from build123d import *

# Parameters (mm, degrees)
SKETCH1_W                     = 80
SKETCH1_H                     = 35
RECTANGLE_BLOCK_EXTRUDE_DEPTH = 45
HOLLOW_OUT_BLOCK_CUT_DEPTH    = 81
OPEN_CORNER_CUT_DEPTH         = 81
TOP_CUTS_REACH                = 37
SKETCH15_R                    = 4
CIRCLE_CUT_ON_FRONT_REACH     = 12
SKETCH18_R                    = 4
RECTANGLE_CUT_ON_BACK_DEPTH   = 5
CUT_EXTRUDE17_DEPTH           = 81
SKETCH25_W                    = 40
SKETCH25_H                    = 3
SKETCH25_H_2                  = 17
CUT_EXTRUDE18_DEPTH           = 10
BOSS_EXTRUDE6_DEPTH           = 5


with BuildPart() as part:
    # Sketch1 → Rectangle Block Extrude (new body)
    with BuildSketch(Plane.XY):
        Rectangle(SKETCH1_W, SKETCH1_H)
    extrude(amount=RECTANGLE_BLOCK_EXTRUDE_DEPTH)

    # Sketch11 → Hollow Out Block Cut (cut, through all)
    with BuildSketch(Plane.ZY.offset(40)):
        with BuildLine():
            Line((8, 12.5), (37, 12.5))
            ThreePointArc((37, 12.5), (39.121320344, 11.621320344), (40, 9.5))
            Line((40, 9.5), (40, -9.5))
            ThreePointArc((40, -9.5), (39.121320344, -11.621320344), (37, -12.5))
            Line((37, -12.5), (8, -12.5))
            ThreePointArc((8, -12.5), (5.878679656, -11.621320344), (5, -9.5))
            Line((5, -9.5), (5, 9.5))
            ThreePointArc((5, 9.5), (5.878679656, 11.621320344), (8, 12.5))
        make_face()
    extrude(amount=-HOLLOW_OUT_BLOCK_CUT_DEPTH, mode=Mode.SUBTRACT)

    # Sketch12 → Open Corner Cut (cut, through all)
    with BuildSketch(Plane.ZY.offset(40)):
        with BuildLine():
            Line((35, 17.5), (35, 12.5))
            Line((35, 12.5), (37, 12.5))
            ThreePointArc((37, 12.5), (39.121320344, 11.621320344), (40, 9.5))
            Line((40, 9.5), (40, 2.5))
            Line((40, 2.5), (45, 2.5))
            Line((45, 2.5), (45, 17.5))
            Line((45, 17.5), (35, 17.5))
        make_face()
    extrude(amount=-OPEN_CORNER_CUT_DEPTH, mode=Mode.SUBTRACT)

    # Sketch15 → Top Cuts (cut, up to next)
    with BuildSketch(Plane(origin=(0, 17.5, 0), x_dir=(1, 0, 0), z_dir=(0, 1, 0)), mode=Mode.PRIVATE) as top_cuts_sk1:
        with BuildLine():
            Line((17, -8), (-17, -8))
            ThreePointArc((-17, -8), (-19.121320344, -8.878679656), (-20, -11))
            Line((-20, -11), (-20, -35))
            Line((-20, -35), (20, -35))
            Line((20, -35), (20, -11))
            ThreePointArc((20, -11), (19.121320344, -8.878679656), (17, -8))
        make_face()
    top_cuts_tool1 = extrude(top_cuts_sk1.sketch, amount=-TOP_CUTS_REACH, mode=Mode.PRIVATE) & part.part
    add(top_cuts_tool1.solids().sort_by_distance((0, 17.5, 21.546053))[0], mode=Mode.SUBTRACT)
    # Sketch15 → Top Cuts (cut, up to next)
    with BuildSketch(Plane(origin=(0, 17.5, 0), x_dir=(1, 0, 0), z_dir=(0, 1, 0)), mode=Mode.PRIVATE) as top_cuts_sk2:
        with Locations((-30, -23)):
            Circle(SKETCH15_R)
    top_cuts_tool2 = extrude(top_cuts_sk2.sketch, amount=-TOP_CUTS_REACH, mode=Mode.PRIVATE) & part.part
    add(top_cuts_tool2.solids().sort_by_distance((-30, 17.5, 23))[0], mode=Mode.SUBTRACT)
    # Sketch15 → Top Cuts (cut, up to next)
    with BuildSketch(Plane(origin=(0, 17.5, 0), x_dir=(1, 0, 0), z_dir=(0, 1, 0)), mode=Mode.PRIVATE) as top_cuts_sk3:
        with Locations((30, -23)):
            Circle(SKETCH15_R)
    top_cuts_tool3 = extrude(top_cuts_sk3.sketch, amount=-TOP_CUTS_REACH, mode=Mode.PRIVATE) & part.part
    add(top_cuts_tool3.solids().sort_by_distance((30, 17.5, 23))[0], mode=Mode.SUBTRACT)

    # Sketch18 → Circle Cut on Front (cut, up to next)
    with BuildSketch(Plane.XY.offset(35), mode=Mode.PRIVATE) as circle_cut_on_front_sk1:
        with Locations((-30, -5.5)):
            Circle(SKETCH18_R)
    circle_cut_on_front_tool1 = extrude(circle_cut_on_front_sk1.sketch, amount=CIRCLE_CUT_ON_FRONT_REACH, mode=Mode.PRIVATE) & part.part
    add(circle_cut_on_front_tool1.solids().sort_by_distance((-30, -5.5, 35))[0], mode=Mode.SUBTRACT)
    # Sketch18 → Circle Cut on Front (cut, up to next)
    with BuildSketch(Plane.XY.offset(35), mode=Mode.PRIVATE) as circle_cut_on_front_sk2:
        with Locations((30, -5.5)):
            Circle(SKETCH18_R)
    circle_cut_on_front_tool2 = extrude(circle_cut_on_front_sk2.sketch, amount=CIRCLE_CUT_ON_FRONT_REACH, mode=Mode.PRIVATE) & part.part
    add(circle_cut_on_front_tool2.solids().sort_by_distance((30, -5.5, 35))[0], mode=Mode.SUBTRACT)

    # Sketch23 → Rectangle Cut on Back (cut)
    with BuildSketch(Plane(origin=(0, 0, 0), x_dir=(-1, 0, 0), z_dir=(0, 0, -1))):
        with BuildLine():
            Line((22, 5.5), (-22, 5.5))
            ThreePointArc((-22, 5.5), (-24.121320344, 4.621320344), (-25, 2.5))
            Line((-25, 2.5), (-25, -2.5))
            ThreePointArc((-25, -2.5), (-24.121320344, -4.621320344), (-22, -5.5))
            Line((-22, -5.5), (22, -5.5))
            ThreePointArc((22, -5.5), (24.121320344, -4.621320344), (25, -2.5))
            Line((25, -2.5), (25, 2.5))
            ThreePointArc((25, 2.5), (24.121320344, 4.621320344), (22, 5.5))
        make_face()
    extrude(amount=-RECTANGLE_CUT_ON_BACK_DEPTH, mode=Mode.SUBTRACT)

    # Sketch24 → Cut-Extrude17 (cut, through all)
    with BuildSketch(Plane.ZY.offset(40)):
        with BuildLine():
            Line((3, -17.5), (0, -17.5))
            Line((0, -17.5), (0, -14.5))
            ThreePointArc((0, -14.5), (0.878679656, -16.621320344), (3, -17.5))
        make_face()
        with BuildLine():
            Line((0, 14.5), (0, 17.5))
            Line((0, 17.5), (3, 17.5))
            ThreePointArc((3, 17.5), (0.878679656, 16.621320344), (0, 14.5))
        make_face()
        with BuildLine():
            Line((42, -17.5), (45, -17.5))
            Line((45, -17.5), (45, -14.5))
            ThreePointArc((45, -14.5), (44.121320344, -16.621320344), (42, -17.5))
        make_face()
    extrude(amount=-CUT_EXTRUDE17_DEPTH, mode=Mode.SUBTRACT)

    # Sketch25 → Cut-Extrude18 (cut)
    with BuildSketch(Plane.XY.offset(45)):
        with Locations((0, -16)):
            Rectangle(SKETCH25_W, SKETCH25_H)
        with Locations((0, -6)):
            Rectangle(SKETCH25_W, SKETCH25_H_2)
    extrude(amount=-CUT_EXTRUDE18_DEPTH, mode=Mode.SUBTRACT)

    # Sketch28 → Boss-Extrude6 (add)
    with BuildSketch(Plane(origin=(0, -17.5, 0), x_dir=(-1, 0, 0), z_dir=(0, -1, 0))):
        with BuildLine():
            Line((-20, -38), (-20, -35))
            Line((-20, -35), (-17, -35))
            ThreePointArc((-17, -35), (-19.121320344, -35.878679656), (-20, -38))
        make_face()
        with BuildLine():
            Line((20, -38), (20, -35))
            Line((20, -35), (17, -35))
            ThreePointArc((17, -35), (19.121320344, -35.878679656), (20, -38))
        make_face()
    extrude(amount=-BOSS_EXTRUDE6_DEPTH)


solid = part.part
Source: CAD feature listing. Evaluate the final solid. Frame: model axes, mm. A direction names the side the tool comes from. Round coordinates to 2 decimals unless told otherwise and drop trailing zeros. Loops run counter-clockwise (first coordinate to the right, second up) from the corner with the lowest first, then second, coordinate; pieces in that order, holes last. Notation, with made-up numbers: (84.25, -4) - (111.25, -4) arc R12 cw to (111.25, 14) - close; hole circle Ø5 at (-35, 1.5). An arc over 180 degrees is marked (long way). Write item = value, one per line. Start each with the question number.
(1) Set-up query: faces 1 (the face through (-20, -7, 42)), 2 (the face through (20, 15, 23)), 3 (the face through (-29, 12.5, 18)). Return all of +Z, -Z, +X, -X, +Y, -Y with unobstructed straight access to the full face (end or side cutting, diameter ignored); none if empty.
(2) Section query D-D, the plane x = -31.5. Output: boundary loops of the cut face in (y, z), plus the area to 3 significant figures.
(3) Pin query (flat end, axial travel): pin 1 (2.5 mm diameter, centred on x = 29, y = 14, fed in from +Z); pin 2 (2 mm diameter, centred on x = 11, z = 29.5, fed in from +Y); pin 3 (5.5 mm diameter, centred on x = 28.5, z = 42.5, fed in from +Y). Return the tip coordinate at first contact, or that it passes through.
(4) Section query B-B, the plane z = 23. Output: boundary loops of the cut face in (x, y), plus the area to 3 significant figures.
(5) Section query C-C, the plane y = -4.5. Output: boundary loops of the cut face in (x, z), plus the area to 3 significant figures.
(6) Pull-direction query (Y, two-part tool) for faces 4 (the face through (40, -13, 19)), 5 (the face through (30, 2.5, 42)), 6 (the face through (0, -5.5, 2)), 7 (the face through (24.1, 4.64, 2.46)); classes: +Y half, -Y half, draft (parallel to the pull), parting line (faces both ways), or undercut.
(7) Section query A-A, the plane x = -7. Output: boundary loops of the cut face in (y, z), plus the area to 3 significant figures.
(8) Ray query, line 1 along X through (y, z) = (13.8, 23); line 2 along Y through (x, z) = (26.5, 25); line 3 along Z through (x, y) = (-16, -13.5). Return the intervals inside material, ascending. Write a range as from..to.
Conclusion:
q1.face_1 = +Z, +Y, -Y
q1.face_2 = +Z, +Y
q1.face_3 = +Z, +X, -X
q2.outline = (-17.5, 3) arc R3 ccw to (-14.5, 0) - (14.5, 0) arc R3 ccw to (17.5, 3) - (17.5, 19.29) - (12.5, 19.29) - (12.5, 8) arc R3 cw to (9.5, 5) - (-9.5, 5) arc R3 cw to (-12.5, 8) - (-12.5, 37) arc R3 cw to (-9.5, 40) - (-9.21, 40) - (-9.21, 45) - (-14.5, 45) arc R3 ccw to (-17.5, 42) - close; (-1.79, 40) - (2.5, 40) - (2.5, 45) - (-1.79, 45) - close; (12.5, 26.71) - (17.5, 26.71) - (17.5, 35) - (12.5, 35) - close
q2.area = 526 mm2
q3.pin_1 = 35
q3.pin_2 = -12.5
q3.pin_3 = 2.5
q4.outline = (-40, -17.5) - (40, -17.5) - (40, -12.5) - (-40, -12.5) - close; (-40, 12.5) - (-34, 12.5) - (-34, 17.5) - (-40, 17.5) - close; (-26, 12.5) - (-20, 12.5) - (-20, 17.5) - (-26, 17.5) - close; (20, 12.5) - (26, 12.5) - (26, 17.5) - (20, 17.5) - close; (34, 12.5) - (40, 12.5) - (40, 17.5) - (34, 17.5) - close
q4.area = 520 mm2
q5.outline = (-40, 0) - (-24.24, 0) - (-24.24, 5) - (-40, 5) - close; (-40, 40) - (-33.87, 40) - (-33.87, 45) - (-40, 45) - close; (-26.13, 40) - (-20, 40) - (-20, 45) - (-26.13, 45) - close; (20, 40) - (26.13, 40) - (26.13, 45) - (20, 45) - close; (24.24, 0) - (40, 0) - (40, 5) - (24.24, 5) - close; (33.87, 40) - (40, 40) - (40, 45) - (33.87, 45) - close
q5.area = 280 mm2
q6.face_4 = draft
q6.face_5 = +Y half
q6.face_6 = undercut
q6.face_7 = undercut
q7.outline = (-17.5, 3) arc R3 ccw to (-14.5, 0) - (-5.5, 0) - (-5.5, 5) - (-9.5, 5) arc R3 cw to (-12.5, 8) - (-12.5, 35) - (-17.5, 35) - close; (5.5, 0) - (14.5, 0) arc R3 ccw to (17.5, 3) - (17.5, 8) - (12.5, 8) arc R3 cw to (9.5, 5) - (5.5, 5) - close
q7.area = 285 mm2
q8.line_1 = -40..-34, -26..-20, 20..26, 34..40
q8.line_2 = -17.5..-12.5, 12.5..17.5
q8.line_3 = 0..35
